For this review, take the finished solid that the model builds, in its own axes (mm). A direction names the side the tool comes from. Round coordinates to 2 decimals unless told otherwise and drop trailing zeros. Write each loop counter-clockwise with the first axis right and the second up, starting at its lowest first coordinate (ties: lowest second). Pieces come first, ordered by that corner, then holes. Notation, with made-up numbers: (62, 1) -> (81, 1) arc R30 cw to (81, 32) -> close; hole circle Ø11 at (-5.5, -29.75). An arc over 180 degrees is marked (long way). Write each question's results on one line, items separated by ' | '. Start each with the question number.
Item 1: The part is to be moulded in two halves that separate along Y. For faces 3 (the cylindrical face through (26.1, -31.5, 2)), 4 (the flat face through (-10.16, 18.34, 1.97)), 5 (the cylindrical face through (-8.697, -70.464, 2.028)), 6 (the cylindrical face through (-8.697, 70.464, 2.028)), say which applies: +Y half, -Y half, draft (parallel to the pull), parting line (faces both ways), or undercut.
Item 2: To check wall thickness, follow line 1 along Y through (x, z) = (-38, 3.85); line 2 along X through (y, z) = (0.5, 2.3); line 3 along Y through (x, z) = (-29, 0.8). State the ranges of each line that lie inside material, in increasing order.
Item 3: Tool access review of faces 1 (the flat face through (27.875, 49.801, 1.972)), 2 (the cylindrical face through (25.9, 31.5, 2)): name each direction out of +Z, -Z, +X, -X, +Y, -Y from which nothing blocks a thin tool from reaching the whole face with its end or side.
Item 4: Add section B-B (z = 2.1). Count the separate pieces of the cut face and the enclosed holes in it, plus the area to 3 significant figures.
Item 5: Clearance check with a flat-ended pin moving along its axis: pin 1 (6 mm diameter, centred on x = -27.5, y = 28, fed in from -Z). State where the tip first meets the part, or that it passes through.
Item 6: Add section C-C (y = 53). State the section outline as (x, z) points, plus the area to 3 significant figures.
Item 7: Add section D-D (x = 56.5). State the section outline as (y, z) points, plus the area to 3 significant figures.
Item 8: Add section A-A (x = 9.5). State the section outline as (y, z) points.
from build123d import *

# Parameters (mm, degrees)
SKETCH_1_R      = 1.6
EXTRUDE_1_DEPTH = 4
FILLET_1_R      = 3


with BuildPart() as part:
    # 草图1 → 凸台-拉伸1 (new body)
    with BuildSketch(Plane.XY):
        Polygon((65.464500341, 28.098076211), (65.464500341, -28.098076211), (-8.718623412, -70.927722679), (-57.385919005, -42.829646468), (-57.385919005, 42.829646468), (-8.718623412, 70.927722679), align=None)
        with Locations((60.964500341, 25.5)):
            Circle(SKETCH_1_R, mode=Mode.SUBTRACT)
        with Locations((60.964500341, -25.5)):
            Circle(SKETCH_1_R, mode=Mode.SUBTRACT)
        with Locations((-8.398602374, -65.546806024)):
            Circle(SKETCH_1_R, mode=Mode.SUBTRACT)
        with Locations((-52.565897967, -40.046806024)):
            Circle(SKETCH_1_R, mode=Mode.SUBTRACT)
        with Locations((-52.565897967, 40.046806024)):
            Circle(SKETCH_1_R, mode=Mode.SUBTRACT)
        with Locations((-8.398602374, 65.546806024)):
            Circle(SKETCH_1_R, mode=Mode.SUBTRACT)
        with BuildLine():
            Line((30.964500341, 26.5), (30.964500341, -26.5))
            ThreePointArc((30.964500341, -26.5), (25.964500341, -31.5), (20.964500341, -26.5))
            Line((20.964500341, -26.5), (20.964500341, 26.5))
            ThreePointArc((20.964500341, 26.5), (25.964500341, 31.5), (30.964500341, 26.5))
        make_face(mode=Mode.SUBTRACT)
        with BuildLine():
            Line((7.46742303, -40.06604391), (-38.431923371, -13.56604391))
            ThreePointArc((-38.431923371, -13.56604391), (-40.26205039, -6.735916892), (-33.431923371, -4.905789873))
            Line((-33.431923371, -4.905789873), (12.46742303, -31.405789873))
            ThreePointArc((12.46742303, -31.405789873), (14.297550049, -38.235916892), (7.46742303, -40.06604391))
        make_face(mode=Mode.SUBTRACT)
        with BuildLine():
            Line((-38.431923371, 13.56604391), (7.46742303, 40.06604391))
            ThreePointArc((7.46742303, 40.06604391), (14.297550049, 38.235916892), (12.46742303, 31.405789873))
            Line((12.46742303, 31.405789873), (-33.431923371, 4.905789873))
            ThreePointArc((-33.431923371, 4.905789873), (-40.26205039, 6.735916892), (-38.431923371, 13.56604391))
        make_face(mode=Mode.SUBTRACT)
    extrude(amount=EXTRUDE_1_DEPTH)

    # 圆角1
    fillet_1_edges = [part.edges().sort_by_distance(p)[0] for p in [
        (-57.385919005, 42.829646468, 2),
        (-8.718623412, 70.927722679, 2),
        (65.464500341, 28.098076211, 2),
        (65.464500341, -28.098076211, 2),
        (-8.718623412, -70.927722679, 2),
        (-57.385919005, -42.829646468, 2),
    ]]
    fillet(fillet_1_edges, radius=FILLET_1_R)


solid = part.part
Responses:
1) face 3: undercut | face 4: undercut | face 5: -Y half | face 6: +Y half
2) line 1: y = -54.02 to -13.82, -4.68 to 4.68, 13.82 to 54.02 | line 2: x = -57.39 to 20.96, 30.96 to 65.46 | line 3: y = -59.22 to -19.01, -7.46 to 7.46, 19.01 to 59.22
3) face 1: +Z, -Z, +X, +Y | face 2: +Z, -Z
4) separate pieces: 1 | enclosed holes: 9 | area: 11,000 mm^2
5) pin 1: stops at z = 0
6) outline: (-39.77, 0) -> (22.33, 0) -> (22.33, 4) -> (-39.77, 4) -> close | area: 248 mm^2
7) outline: (-33.27, 0) -> (33.27, 0) -> (33.27, 4) -> (-33.27, 4) -> close | area: 266 mm^2
8) outline: (-60.41, 0) -> (-40.71, 0) -> (-40.71, 4) -> (-60.41, 4) -> close; (-29.69, 0) -> (29.69, 0) -> (29.69, 4) -> (-29.69, 4) -> close; (40.71, 0) -> (60.41, 0) -> (60.41, 4) -> (40.71, 4) -> close
